For this review, take the finished solid that the model builds, in its own axes (mm). A direction names the side the tool comes from. Give positions to 0.01 mm unless a question says otherwise; leave off trailing zeros. Order: outer loops, then holes, each group sorted by start corner. A loop starts at its lowest first (then second) coordinate and runs counter-clockwise, first axis right, second up. Notation, with made-up numbers: M -31,-27.5 L -6,-27.5 A18 cw -6,-1.5 Z; hole C -36.75,-38 d1. An arc over 180 degrees is marked long. Use CSV: the item, a comma, the result in double quotes. Start each with the question number.
(1) Clearance check with flat-ended pins moving along their axes: P1, Ø2, axis at x = 23, z = -4, coming from the +Y side; P2, Ø3, axis at x = 22, y = 3.5, coming from the -Z side; P3, Ø4, axis at x = 5.5, z = 3, coming from the +Y side. State where each tip first meets the part, or that it passes through.
(2) Consider section A-A (z = 0). Write out the cut boundary in (x, y).
(3) Consider section D-D (y = -4.5). Write out the cut boundary in (x, z).
(4) Consider section C-C (x = 19). Write out the cut boundary in (y, z), and give its area (3 significant figures).
(5) Consider section B-B (y = -1.5). Write out the cut boundary in (x, z).
(6) Wall thickness on L1, parallel to X at y = 4.75, z = 4; L2, parallel to Y at x = 6, z = -3; L3, parallel to Z at x = 35.5, y = -0.5: over which ranges is each line inside the solid? List them lowest first. Write a range as from..to.
(7) Tool access review of faces 1 (the face through (19.317, -0.867, -3.905)), 2 (the face through (39.62, -3.15, 5.83)): name each direction out of +Z, -Z, +X, -X, +Y, -Y from which nothing blocks a thin tool from reaching the whole face with its end or side.
Autodesk Inventor part; units mm, degrees
ref_plane "YZ Plane" through (0, 0, 0) normal (1, 0, 0) x (0, 1, 0)
ref_plane "XZ Plane" through (0, 0, 0) normal (0, 1, 0) x (-1, 0, 0)
ref_plane "XY Plane" through (0, 0, 0) normal (0, 0, 1) x (1, 0, 0)
sketch "Sketch1" plane through (0, 0, 0) normal (0, 0, 1) x (1, 0, 0)
  line L0 (0, 0) -> (0, 4)
  line L1 (0, 4) -> (38.1, 4)
  line L2 (38.1, 4) -> (38.1, 7.5)
  line L3 (38.1, 7.5) -> (41.1, 7.5)
  line L4 (41.1, 7.5) -> (41.1, 0)
  line L5 (41.1, 0) -> (0, 0)
  dimension "d0" = 4
  dimension "d1" = 38.1
  dimension "d2" = 3
  dimension "d3" = 7.5
revolve "Revolution1" add sketch "Sketch1" angle 360 about axis through (41.1, 0, 0) along (-1, 0, 0)
sketch "Sketch2" plane through (41.1, 0, 0) normal (1, 0, 0) x (0, 0, -1)
  circle A0 centre (0, 0) radius 7.5
  line L0 (-4.212, 6.2056) -> (4.212, 6.2056)
  line L1 (7.5, 0) -> (4.212, 6.2056)
  line L2 (7.5, 0) -> (4.212, -6.2056)
  line L3 (4.212, -6.2056) -> (-4.212, -6.2056)
  line L4 (-4.212, -6.2056) -> (-7.5, 0)
  line L5 (-4.212, 6.2056) -> (-7.5, 0)
extrude "Extrusion1" cut sketch "Sketch2" against normal up to next contours L1 A0 | A0 L2 | L0 A0 | A0 L3 | L5 A0 | A0 L4
properties part number "8mm_x_rail_connection"
Check result:
1,P1,"stops at y = 2.65"
1,P2,"stops at z = -3.46"
1,P3,"stops at y = 3.87"
2,outline,"M 0,-4 L 38.1,-4 L 38.1,-6.21 L 41.1,-6.21 L 41.1,6.21 L 38.1,6.21 L 38.1,4 L 0,4 Z"
3,outline,"M 38.1,-5.12 L 41.1,-5.12 L 41.1,5.12 L 38.1,5.12 Z"
4,outline,"C 0,0 d8"
4,area,"50.3 mm^2"
5,outline,"M 0,-3.71 L 38.1,-3.71 L 38.1,-6.71 L 41.1,-6.71 L 41.1,6.71 L 38.1,6.71 L 38.1,3.71 L 0,3.71 Z"
6,L1,"x = 38.1..41.1"
6,L2,"y = -2.65..2.65"
6,L3,"z = -3.97..3.97"
7,face 1,"-X"
7,face 2,"+Z, +X, -X, -Y"
